```python
from build123d import *

# Parameters (mm, degrees)
SKETCH1_R           = 1.5
BOSS_EXTRUDE1_DEPTH = 6
FILLET2_R           = 5


with BuildPart() as part:
    # Sketch1 → Boss-Extrude1 (new body)
    with BuildSketch(Plane.XY):
        with BuildLine():
            Line((19.944251464, 5), (0, 5))
            ThreePointArc((0, 5), (-5, 0), (0, -5))
            Line((0, -5), (22, -5))
            ThreePointArc((22, -5), (22.969031552, -4.905199063), (23.901317064, -4.624391141))
            Line((23.901317064, -4.624391141), (25.223175743, -5.70274446))
            Line((25.223175743, -5.70274446), (25.404244184, -4.006463095))
            Line((25.404244184, -4.006463095), (26.726102864, -5.084816415))
            Line((26.726102864, -5.084816415), (26.907171305, -3.388535049))
            Line((26.907171305, -3.388535049), (28.229029985, -4.466888369))
            Line((28.229029985, -4.466888369), (28.410098426, -2.770607004))
            Line((28.410098426, -2.770607004), (29.731957105, -3.848960323))
            Line((29.731957105, -3.848960323), (29.913025547, -2.152678958))
            ThreePointArc((29.913025547, -2.152678958), (38.729983808, 7.959751364), (52.110103023, 6.973642948))
            Line((52.110103023, 6.973642948), (53.431961702, 5.895289628))
            Line((53.431961702, 5.895289628), (53.613030144, 7.591570993))
            Line((53.613030144, 7.591570993), (54.934888823, 6.513217674))
            Line((54.934888823, 6.513217674), (55.115957264, 8.209499039))
            Line((55.115957264, 8.209499039), (56.437815944, 7.13114572))
            Line((56.437815944, 7.13114572), (56.618884385, 8.827427085))
            Line((56.618884385, 8.827427085), (57.940743065, 7.749073765))
            Line((57.940743065, 7.749073765), (58.121811506, 9.44535513))
            Line((58.121811506, 9.44535513), (56.143278706, 14.257550701))
            Line((56.143278706, 14.257550701), (36.302637348, 16.436961709))
            Line((36.302637348, 16.436961709), (19.944251464, 5))
        make_face()
        Circle(SKETCH1_R, mode=Mode.SUBTRACT)
        with Locations((22, 0)):
            Circle(SKETCH1_R, mode=Mode.SUBTRACT)
        with Locations((37.054498685, 12.034873136)):
            Circle(SKETCH1_R, mode=Mode.SUBTRACT)
    extrude(amount=BOSS_EXTRUDE1_DEPTH)

    # Fillet2
    fillet2_edges = [part.edges().sort_by_distance(p)[0] for p in [
        (19.944251464, 5, 3),
        (36.302637348, 16.436961709, 3),
        (56.143278706, 14.257550701, 3),
    ]]
    fillet(fillet2_edges, radius=FILLET2_R)


solid = part.part
```
Can you work these out from the model? Positions are in its coordinate system, mm. A direction names the side the tool comes from. Coordinates: 2 decimals unless noted, no trailing zeros. Loops run counter-clockwise (first coordinate to the right, second up) from the corner with the lowest first, then second, coordinate; pieces in that order, holes last.
Item 1: Please list where these lines run through material, in increasing order: L1, parallel to X at y = 7, z = 1.4; L2, parallel to X at y = 6.75, z = 4; L3, parallel to Y at x = 0, z = 2.7.
Answers below:
L1: x = 22.8 to 36.8, 52.07 to 53.55, 54.34 to 54.99
L2: x = 22.45 to 36.39, 52.38 to 53.52, 54.64 to 54.96
L3: y = -5 to -1.5, 1.5 to 5
Item 2: Suppose I cut it at A-A (y = 0). Please give me the cut outline in (x, z).
Answers below:
outline: (-5, 0) - (-1.5, 0) - (-1.5, 6) - (-5, 6) - close; (1.5, 0) - (20.5, 0) - (20.5, 6) - (1.5, 6) - close; (23.5, 0) - (30.65, 0) - (30.65, 6) - (23.5, 6) - close
Item 3: I'm going to push flat-ended pins straight in: pin 1 (12 mm diameter, centred on x = 4, y = 7, fed in from -Z); pin 2 (1.5 mm diameter, centred on y = 8, z = 5, fed in from -X); pin 3 (1.8 mm diameter, centred on x = 12, z = 3.5, fed in from -Y); pin 4 (2.5 mm diameter, centred on x = 37.05, y = 12.03, fed in from +Z). Where does each tip first touch, or does it pass through?
Answers below:
pin 1: stops at z = 0
pin 2: stops at x = 23.16
pin 3: stops at y = -5
pin 4: passes through
Item 4: Suppose I cut it at B-B (z = 1.5). State how many separate pieces and enclosed holes the cut face has, then the cut area to 3 significant figures.
Answers below:
separate pieces: 1
enclosed holes: 3
area: 565 mm2
Item 5: Which directions (+Z, -Z, +X, -X, +Y, -Y) give clear straight access to the entire face, cutting with the end or side of a thin tool? Please do faces 5 (the face through (38.55, 7.885, 2.958)), 6 (the face through (9, 5, 3)).
Answers below:
face 5: +Z, -Z, -Y
face 6: +Z, -Z, -X, +Y
Item 6: If we mould it in two halves opening along X, with no side actions, what happens to faces 1 (the face through (56.527, 7.967, 2.958)), 2 (the face through (-5, 0, 3)), 3 (the face through (45.788, 15.395, 2.958)), 4 (the face through (11, -5, 3))? For each: released by +X, released by -X, zero draft, split by the parting line, or undercut.
Answers below:
face 1: undercut
face 2: released by -X
face 3: released by +X
face 4: zero draft
Item 7: Suppose I cut it at C-C (x = 17.5). Please give me the cut outline in (y, z).
Answers below:
outline: (-5, 0) - (5, 0) - (5, 6) - (-5, 6) - close
